Build history of the part. All positions in model axes, mm. A direction names the side the tool comes from. Give positions to 0.01 mm unless a question says otherwise; leave off trailing zeros. Write each loop counter-clockwise with the first axis right and the second up, starting at its lowest first coordinate (ties: lowest second). Pieces come first, ordered by that corner, then holes. Notation, with made-up numbers: M -30.5,53.25 L 28.5,53.25 A12 ccw 28.5,65.25 Z; hole C 11,75.5 d3. An arc over 180 degrees is marked long. Return JSON: item names as keys, results as strings. Group by question number.
Q1. Band-saw the part on C-C, the plane z = 4. Give the cut face in (x, y) (3 decimals), then the cut area to 3 significant figures.
Q2. Band-saw the part on A-A, the plane y = 0.25. Give the cut face in (x, z) (3 decimals).
Q3. Flat gauge pins, fed straight in: pin 1 Ø4 at (x, y) = (264.5, 3.5) entering from +Z (3 decimals); pin 2 Ø8 at (y, z) = (6.5, -17) entering from -X. Where does each tip first touch, or does it go through?
Q4. Tool access for faces 4 (the flat face through (202, 1, 22.225)), 5 (the flat face through (116.294, -11.23, 0.119)): list every direction of +Z, -Z, +X, -X, +Y, -Y with a clear straight run to the whole face (end or side of a thin tool).
Q5. Pull direction Z, two halves, no side cores. Call faces 1 (the flat face through (202, 0, 25.4)), 2 (the flat face through (202, -9.525, -5)), 3 (the flat face through (201, -12.7, -5)): +Z half, -Z half, draft (parallel to the pull), parting line (faces both ways), or undercut.
Q6. Band-saw the part on D-D, the plane x = 277. Give the cut face in (y, z) (3 decimals), then the cut area to 3 significant figures.
Q7. Wall check: probe 1 along Z at (x, y) = (190, 2.25) (3 decimals); probe 2 along Y at (x, z) = (306, -13.5) (3 decimals); probe 3 along Z at (x, y) = (270, 0.5) (3 decimals). Give the ranges that are in metal, low to high.
Q8. Band-saw the part on B-B, the plane x = 104.5. Give the cut face in (y, z) (3 decimals), then the cut area to 3 significant figures.
from build123d import *

# Parameters (mm, degrees)
BOSS_EXTRUDE1_DEPTH = 406.4
CUT_EXTRUDE1_DEPTH  = 408.984411467


with BuildPart() as part:
    # Sketch1 → Boss-Extrude1 (new body)
    with BuildSketch(Plane(origin=(0, 0, 0), x_dir=(0, 0, -1), z_dir=(1, 0, 0))):
        Polygon((-22.225, -9.525), (-22.225, 12.7), (-25.4, 12.7), (-25.4, -12.7), (25.4, -12.7), (25.4, 12.7), (22.225, 12.7), (22.225, -9.525), align=None)
    extrude(amount=BOSS_EXTRUDE1_DEPTH)

    # Sketch2 → Cut-Extrude1 (cut, through all)
    with BuildSketch(Plane(origin=(0, 12.7, 0), x_dir=(1, 0, 0), z_dir=(0, 1, 0))):
        Polygon((203.2, -25.4), (152.4, -25.4), (79.850081258, 25.4), (-62.210264403, 25.4), (-62.210264403, -94.274139353), (523.373076947, -141.453594379), (523.373076947, 25.4), (326.549918742, 25.4), (254, -25.4), align=None)
    extrude(amount=-CUT_EXTRUDE1_DEPTH, mode=Mode.SUBTRACT)


solid = part.part
From the geometry:
{
 "1": {"outline": "M 121.838,-12.7 L 284.562,-12.7 L 284.562,-9.525 L 121.838,-9.525 Z", "area": "517 mm^2"},
 "2": {"outline": "M 79.85,-25.4 L 326.55,-25.4 L 322.016,-22.225 L 84.384,-22.225 Z; M 147.866,22.225 L 258.534,22.225 L 254,25.4 L 152.4,25.4 Z"},
 "3": {"pin 1": "stops at z = -22.225", "pin 2": "passes through"},
 "4": {"face 4": "+X, -X, +Y", "face 5": "+Z, -X, +Y, -Y"},
 "5": {"face 1": "+Z half", "face 2": "undercut", "face 3": "draft"},
 "6": {"outline": "M -12.7,-25.4 L 12.7,-25.4 L 12.7,-22.225 L -9.525,-22.225 L -9.525,9.295 L -12.7,9.295 Z", "area": "181 mm^2"},
 "7": {"probe 1": "z = -25.4 to -22.225, 22.225 to 25.4", "probe 2": "y = -12.7 to -9.525", "probe 3": "z = -25.4 to -22.225"},
 "8": {"outline": "M -12.7,-25.4 L 12.7,-25.4 L 12.7,-22.225 L -9.525,-22.225 L -9.525,-8.14 L -12.7,-8.14 Z", "area": "125 mm^2"}
}
